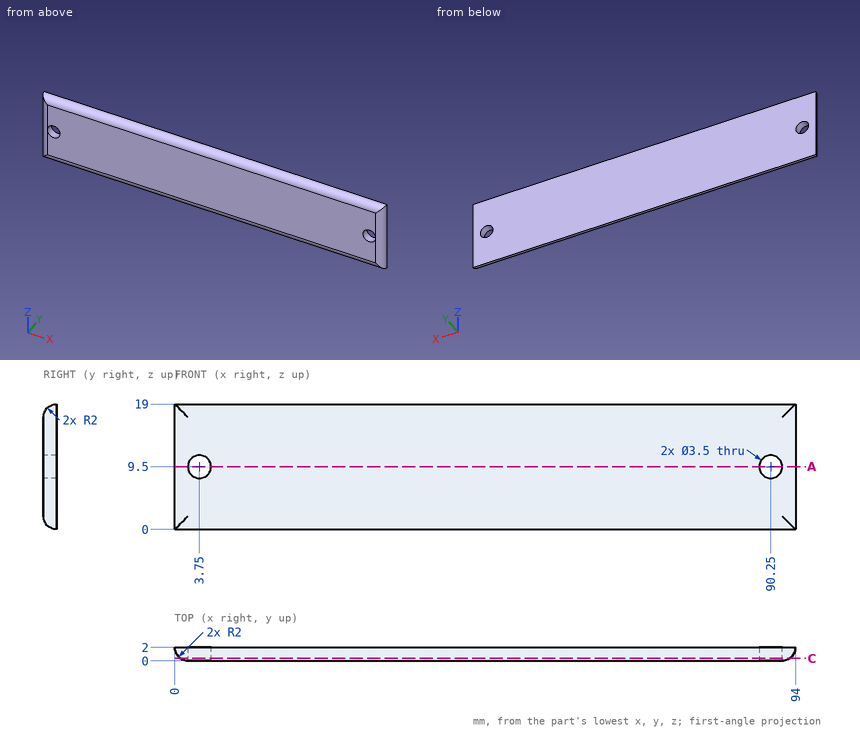
Can you work these out from the drawing? Everything is in mm from the part's minimum corner. Round coordinates to 2 decimals unless told otherwise and drop trailing zeros. Write each loop counter-clockwise with the first axis right and the second up, starting at its lowest first coordinate (ties: lowest second). Pieces come first, ordered by that corner, then holes.
1. Suppose I cut it at A-A (z = 9.5). State how many separate pieces and enclosed holes the cut face has, and give its area (3 significant figures).
2. I need wall thicknesses on L1, parallel to Y at x = 46.5, z = 1.75 (1 decimal); L2, parallel to Z at x = 3.75, y = 1.15; L3, parallel to X at y = 0.5, z = 9.25 (1 decimal). Which ranges of each line are inside material? Lowest first, please.
3. Suppose I cut it at C-C (y = 0.35). List the corners of the cut face in (x, z) for me, and give its area (3 significant figures).
4. Will these pins go through, and if not, where does the flat tip stop? pin 1 Ø1 at (x, y) = (49.5, 1.5) entering from -Z; pin 2 Ø1 at (y, z) = (0.5, 6.5) entering from +X.
Answer sheet:
1. separate pieces: 3
1. enclosed holes: 0
1. area: 172 mm2
2. L1: y = 0 to 2
2. L2: z = 0.19 to 7.75, 11.25 to 18.81
2. L3: x = 0.7 to 2, 5.5 to 88.5, 92 to 93.3
3. outline: (0.87, 0.87) - (93.13, 0.87) - (93.13, 18.13) - (0.87, 18.13) - close; hole circle Ø3.5 at (3.75, 9.5); hole circle Ø3.5 at (90.25, 9.5)
3. area: 1,570 mm2
4. pin 1: stops at z = 0
4. pin 2: stops at x = 93.73
